Could you check a few things on this model? Use its own coordinates, in mm. A direction names the side the tool comes from. Round coordinates to 2 decimals unless told otherwise and drop trailing zeros. Loops run counter-clockwise (first coordinate to the right, second up) from the corner with the lowest first, then second, coordinate; pieces in that order, holes last. Notation, with made-up numbers: M 56,74 L 101,74 A30 cw 101,112 Z; hole C 14,17 d6. An arc over 180 degrees is marked long. One line per item, written item: value. Start each with the question number.
Q1. Imagine slicing it at B-B (z = 33). Please give me the cut outline in (x, y) (3 decimals), then the cut area to 3 significant figures.
Q2. Which directions (+Z, -Z, +X, -X, +Y, -Y) give clear straight access to the entire face, cutting with the end or side of a thin tool? Please do faces 4 (the face through (3.64, 23.88, 43.83)), 5 (the face through (-3.592, 24.558, 43.828)), 6 (the face through (0.094, -4.362, 77.695)), 7 (the face through (-3, 22, 0)).
Q3. Thinking about a two-plate mould opening in Z: for faces 1 (the face through (-0.902, 51.139, 43.828)), 2 (the face through (-3, 22, 88.9)), 3 (the face through (3.599, 13.195, 41.825)), which applies, released by +Z, released by -Z, zero draft, split by the parting line, or undercut?
Q4. Imagine slicing it at D-D (y = 38). Please give me the cut outline in (x, z), then the cut area to 3 significant figures.
Q5. I'm going to push flat-ended pins straight in: pin 1 Ø6 at (x, y) = (0, 10) entering from -Z; pin 2 Ø4 at (y, z) = (19, 50) entering from +X; pin 3 Ø4 at (y, z) = (16.5, 67) entering from +X; pin 4 Ø4 at (x, z) = (-3.5, 38.5) entering from -Y. Where does each tip first touch, or does it pass through?
Q6. Please list where these lines run through material, in increasing order: line 1 along X through (y, z) = (43.5, 5.5); line 2 along X through (y, z) = (48, 9); line 3 along Z through (x, y) = (-4, -1.5).
Q7. Imagine slicing it at C-C (z = 54). Please give me the cut outline in (x, y) (3 decimals).
from build123d import *

# Parameters (mm, degrees)
F1_DEPTH = 88.9
F3_DEPTH = 1.27
F5_DEPTH = 1.27
F6_SIZE  = 1.26999
F8_DEPTH = 12.7


# Not quite as in the source:
# - a fillet or chamfer is up to 0.001 mm smaller than in the source, because OpenCascade refuses the exact size


with BuildPart() as f1:
    # F0 (on Top) → F1 (new body)
    with BuildSketch(Plane.XY):
        with BuildLine():
            Line((-4.064, 0), (-0.635, 48.26))
            ThreePointArc((-0.635, 48.26), (-0.9122099758, 51.1784184141), (-2.1235503767, 53.848))
            ThreePointArc((-2.1235503767, 53.848), (-3.0047663986, 54.0209402292), (-3.1777066278, 53.1397242074))
            ThreePointArc((-3.1777066278, 53.1397242074), (-2.1394148555, 50.8515114195), (-1.9018063048, 48.3500099217))
            Line((-1.9018063048, 48.3500099217), (-5.3308063048, 0.0900099217))
            ThreePointArc((-5.3308063048, 0.0900099217), (0, -5.633003484), (5.3308063048, 0.0900099217))
            Line((5.3308063048, 0.0900099217), (1.9018063048, 48.3500099217))
            ThreePointArc((1.9018063048, 48.3500099217), (2.1394148555, 50.8515114195), (3.1777066278, 53.1397242074))
            ThreePointArc((3.1777066278, 53.1397242074), (3.0047663986, 54.0209402292), (2.1235503767, 53.848))
            ThreePointArc((2.1235503767, 53.848), (0.9122099758, 51.1784184141), (0.635, 48.26))
            Line((0.635, 48.26), (4.064, 0))
            ThreePointArc((4.064, 0), (0, -4.363003484), (-4.064, 0))
        make_face()
    extrude(amount=F1_DEPTH)

    # F2 (on face) → F3 (join)
    with BuildSketch(Plane.XY.offset(88.9)):
        Polygon((-0.3550842778, 34.2804189145), (-1.6218905827, 34.3704288362), (-1.8919203477, 30.5700099217), (-0.6251140428, 30.48), align=None)
        Polygon((0.6251140428, 30.48), (1.8919203477, 30.5700099217), (1.6218905827, 34.3704288362), (0.3550842778, 34.2804189145), align=None)
    extrude(amount=-F3_DEPTH)

    # F4 (on face) → F5 (join)
    with BuildSketch(Plane(origin=(0, 0, 0), x_dir=(1, 0, 0), z_dir=(0, 0, -1))):
        Polygon((-0.6251140428, -30.48), (-1.8919203477, -30.5700099217), (-1.6218905827, -34.3704288362), (-0.3550842778, -34.2804189145), align=None)
        Polygon((1.6218905827, -34.3704288362), (1.8919203477, -30.5700099217), (0.6251140428, -30.48), (0.3550842778, -34.2804189145), align=None)
    extrude(amount=-F5_DEPTH)

    # F6 (size 1.27 in the source; OpenCascade refuses exactly that, so slightly less here)
    f6_edges = [f1.edges().sort_by_distance(p)[0] for p in [
        (-0.490099, 32.380209, 1.27),
        (0.490099, 32.380209, 1.27),
        (-0.490099, 32.380209, 87.63),
        (0.490099, 32.380209, 87.63),
    ]]
    chamfer(f6_edges, length=F6_SIZE)

    # F7 (on Right) → F8 (cut, symmetric)
    with BuildSketch(Plane.YZ):
        with BuildLine():
            ThreePointArc((-5.842, 19.8251978841), (13.3307116053, 44.45), (-5.842, 69.0748021159))
            Line((-5.842, 69.0748021159), (-5.842, 19.8251978841))
        make_face()
    extrude(amount=F8_DEPTH, both=True, mode=Mode.SUBTRACT)


solid = f1.part
Report:
1. outline: M -4.584,10.604 L -3.311,10.604 L -0.635,48.26 A8.89 ccw -2.124,53.848 A0.635 ccw -3.178,53.14 A7.62 cw -1.902,48.35 Z; M 0.635,48.26 L 3.311,10.604 L 4.584,10.604 L 1.902,48.35 A7.62 cw 3.178,53.14 A0.635 ccw 2.124,53.848 A8.89 ccw Z
1. area: 111 mm²
2. face 4: +Z, -Z, +X
2. face 5: +Z, -Z, -X
2. face 6: +Z, -Z
2. face 7: -Z, +X, -X, +Y, -Y
3. face 1: zero draft
3. face 2: released by +Z
3. face 3: undercut
4. outline: M -2.64,0 L -1.36,0 L -1.36,88.9 L -2.64,88.9 Z; M 1.36,0 L 2.64,0 L 2.64,88.9 L 1.36,88.9 Z
4. area: 226 mm²
5. pin 1: passes through
5. pin 2: stops at x = 4.13
5. pin 3: stops at x = 4.31
5. pin 4: stops at y = 12.05
6. line 1: x = -2.25 to -0.97, 0.97 to 2.25
6. line 2: x = -1.93 to -0.65, 0.65 to 1.93
6. line 3: z = 0 to 21.35, 67.55 to 88.9
7. outline: M -4.522,11.467 L -3.249,11.467 L -0.635,48.26 A8.89 ccw -2.124,53.848 A0.635 ccw -3.178,53.14 A7.62 cw -1.902,48.35 Z; M 0.635,48.26 L 3.249,11.467 L 4.522,11.467 L 1.902,48.35 A7.62 cw 3.178,53.14 A0.635 ccw 2.124,53.848 A8.89 ccw Z
